```python
from build123d import *

# Parameters (mm, degrees)
BOSS_EXTRUDE1_DEPTH     = 25
SKETCH2_W               = 40
SKETCH2_H               = 9
BOSS_EXTRUDE2_DEPTH     = 8.18
FILLET1_R               = 5
CUT_EXTRUDE1_DEPTH      = 45.172054958
CUT_EXTRUDE1_DEPTH_BACK = 45.172054958
SKETCH3_R               = 1.5
SKETCH3_3_R             = 3.75
CUT_EXTRUDE2_DEPTH      = 45.172054958
SKETCH4_R               = 1.5
CUT_EXTRUDE3_DEPTH      = 48.026142101
CUT_EXTRUDE9_START      = -9
SKETCH4_4_R             = 4
CUT_EXTRUDE9_DEPTH      = 39.026142101


with BuildPart() as part:
    # Sketch1 → Boss-Extrude1 (new body)
    with BuildSketch(Plane(origin=(0, 0, 0), x_dir=(1, 0, 0), z_dir=(0, 1, 0))):
        with BuildLine():
            Line((0, 0), (-5.555, 0))
            Line((-5.555, 0), (-5.555, 11.82))
            Line((-5.555, 11.82), (15.89, 11.82))
            Line((15.89, 11.82), (34.445, 11.82))
            Line((34.445, 11.82), (34.445, 0))
            Line((34.445, 0), (28.89, 0))
            add(Edge.make_bspline(
                [(0, 0), (14.445, 15.64), (28.89, 0)],
                knots=[0, 0, 0, 1, 1, 1], degree=2))
        make_face()
    extrude(amount=BOSS_EXTRUDE1_DEPTH)

    # Sketch2 → Boss-Extrude2 (add)
    with BuildSketch(Plane(origin=(0, 0, -11.82), x_dir=(-1, 0, 0), z_dir=(0, 0, -1))):
        with Locations((-14.445, 20.5)):
            Rectangle(SKETCH2_W, SKETCH2_H)
    extrude(amount=BOSS_EXTRUDE2_DEPTH)

    # Fillet1
    fillet1_edges = [part.edges().sort_by_distance(p)[0] for p in [
        (14.445, 16, -11.82),
    ]]
    fillet(fillet1_edges, radius=FILLET1_R)

    # Sketch3 → Cut-Extrude1 (cut, two sides: drawn at the far end of the back side and taken through both)
    with BuildSketch(Plane(origin=(0, 0, -11.82), x_dir=(-1, 0, 0), z_dir=(0, 0, -1)).offset(-CUT_EXTRUDE1_DEPTH_BACK)):
        with Locations((-10.445, 4)):
            Circle(SKETCH3_R)
        with Locations((-18.445, 12)):
            Circle(SKETCH3_R)
    extrude(amount=CUT_EXTRUDE1_DEPTH + CUT_EXTRUDE1_DEPTH_BACK, mode=Mode.SUBTRACT)

    # Sketch3<3> → Cut-Extrude2 (cut, through all)
    with BuildSketch(Plane(origin=(0, 0, -11.82), x_dir=(-1, 0, 0), z_dir=(0, 0, -1))):
        with Locations((-18.445, 12)):
            Circle(SKETCH3_3_R)
    extrude(amount=CUT_EXTRUDE2_DEPTH, mode=Mode.SUBTRACT)

    # Sketch4 → Cut-Extrude3 (cut, through all)
    with BuildSketch(Plane(origin=(0, 25, 0), x_dir=(1, 0, 0), z_dir=(0, 1, 0))):
        with Locations(Location((26.445, 16, 0), (0, 0, 270))):
            Circle(SKETCH4_R)
        with Locations(Location((2.445, 16, 0), (0, 0, 270))):
            Circle(SKETCH4_R)
    extrude(amount=-CUT_EXTRUDE3_DEPTH, mode=Mode.SUBTRACT)

    # Sketch4<4> → Cut-Extrude9 (cut, through all)
    with BuildSketch(Plane(origin=(0, 25, 0), x_dir=(1, 0, 0), z_dir=(0, 1, 0)).offset(CUT_EXTRUDE9_START)):
        with Locations((26.445, 16)):
            Circle(SKETCH4_4_R)
        with Locations((2.445, 16)):
            Circle(SKETCH4_4_R)
    extrude(amount=-CUT_EXTRUDE9_DEPTH, mode=Mode.SUBTRACT)


solid = part.part
```
Read the model definition and answer for the solid it produces. Units are mm, in the model's axes. Give positions to 0.01 mm unless a question says otherwise; leave off trailing zeros. Write each loop counter-clockwise with the first axis right and the second up, starting at its lowest first coordinate (ties: lowest second). Pieces come first, ordered by that corner, then holes. Notation, with made-up numbers: M 83,60 L 119,60 A22 ccw 119,68 Z; hole C 44.25,26.5 d9. An arc over 180 degrees is marked long. Put each result on its own line as item: value. Start each with the question number.
1. Each of these flat-tipped pins is pushed along its axis until it touches: pin 1 Ø12 at (x, z) = (17, -7.5) entering from -Y; pin 2 Ø6.5 at (x, z) = (2.445, -16) entering from -Y; pin 3 Ø2.5 at (x, z) = (19.5, -15.5) entering from -Y; pin 4 Ø1 at (x, z) = (10, -13) entering from -Y. Where does it stop, or does it pass through?
2. The part is cut by section B-B, the plane x = -0.5. Give the vertices of the cut face in (y, z), and give its area (3 significant figures).
3. The part is cut by section A-A, the plane z = -16. Give the vertices of the cut face in (x, y) (3 decimals).
4. For a pull along X with two mould halves and no side action, classify faces 1 (the flat face through (34.445, 15, -8)), 2 (the flat face through (15, 16, -17)), 3 (the flat face through (15, 0, -8)) as released by +X, released by -X, zero draft, split by the parting line, or undercut.
5. The part is cut by section D-D, the plane y = 16.75. Give the number of separate pieces and of enclosed holes in the cut face, and give its area (3 significant figures).
6. Consider line 1 along X through (y, z) = (19.25, -16) (3 decimals); line 2 along Y through (x, z) = (18.5, -7.5); line 3 along Z through (x, y) = (27, 20.5). Determine where each line is inside the solid, lowest interval first.
Final values:
1. pin 1: stops at y = 0
1. pin 2: stops at y = 16
1. pin 3: stops at y = 15.37
1. pin 4: stops at y = 13.52
2. outline: M 0,-11.82 L 11,-11.82 A5 cw 14.54,-13.29 L 16,-13.29 L 16,-20 L 25,-20 L 25,0 L 0,0 Z
2. area: 373 mm²
3. outline: M -5.555,15.932 L -1.555,15.932 L -1.555,16 L 0.945,16 L 0.945,25 L -5.555,25 Z; M 3.945,16 L 6.445,16 L 6.445,15.932 L 22.445,15.932 L 22.445,16 L 24.945,16 L 24.945,25 L 3.945,25 Z; M 27.945,16 L 30.445,16 L 30.445,15.932 L 34.445,15.932 L 34.445,25 L 27.945,25 Z
4. face 1: released by +X
4. face 2: undercut
4. face 3: zero draft
5. separate pieces: 1
5. enclosed holes: 2
5. area: 635 mm²
6. line 1: x = -5.555 to 0.945, 3.945 to 24.945, 27.945 to 34.445
6. line 2: y = 0 to 10.5, 13.5 to 25
6. line 3: z = -20 to -17.39, -14.61 to -1.91
